Can you work these out from the drawing? Everything is in mm from the part's minimum corner. Give positions to 0.01 mm unless a question says otherwise; leave off trailing zeros. Order: outer loops, then holes, each group sorted by start corner. A loop starts at its lowest first (then second) coordinate and runs counter-clockwise, first axis right, second up. Notation, with made-up numbers: (-2.75, 45) - (53.25, 45) arc R10 ccw to (53.25, 50) - close; hole circle Ø2 at (-23.75, 0.5). An arc over 180 degrees is marked (long way). One line per question, with ' | ' between items.
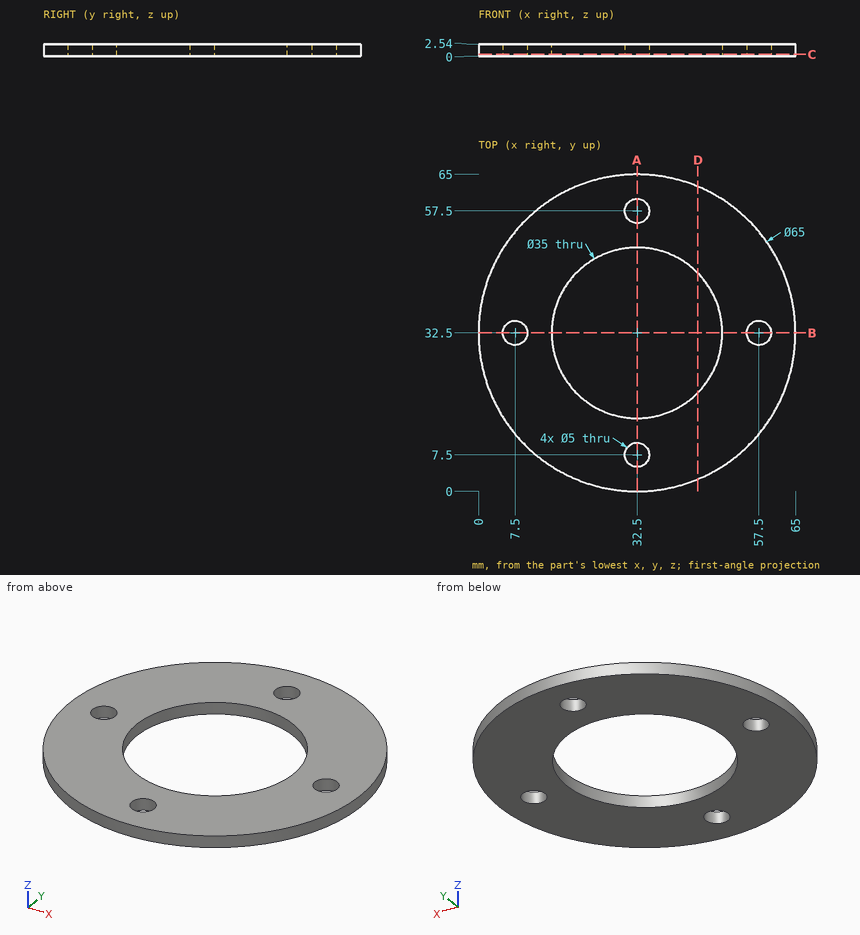
1) Please list where these lines run through material, in increasing order: L1, parallel to Y at x = 32.5, z = 2.05; L2, parallel to Y at x = 30.5, z = 1.65; L3, parallel to Y at x = 57.5, z = 0.55.
Model answer:
L1: y = 0 to 5, 10 to 15, 50 to 55, 60 to 65 | L2: y = 0.06 to 6, 9 to 15.11, 49.89 to 56, 59 to 64.94 | L3: y = 11.73 to 30, 35 to 53.27
2) I'm going to push a flat-ended pin straight in: P1, Ø1.5, axis at x = 39.5, z = 1.5, coming from the +Y side. Where does the tip first touch, or does it pass through?
Model answer:
P1: stops at y = 64.39
3) I want a section at A-A (x = 32.5). List the corners of the cut face in (y, z) for me, plus the area to 3 significant figures.
Model answer:
outline: (0, 0) - (5, 0) - (5, 2.54) - (0, 2.54) - close; (10, 0) - (15, 0) - (15, 2.54) - (10, 2.54) - close; (50, 0) - (55, 0) - (55, 2.54) - (50, 2.54) - close; (60, 0) - (65, 0) - (65, 2.54) - (60, 2.54) - close | area: 50.8 mm2
4) I want a section at C-C (z = 0.4). List the corners of the cut face in (x, y) for me.
Model answer:
outline: circle Ø65 at (32.5, 32.5); hole circle Ø5 at (7.5, 32.5); hole circle Ø35 at (32.5, 32.5); hole circle Ø5 at (32.5, 7.5); hole circle Ø5 at (32.5, 57.5); hole circle Ø5 at (57.5, 32.5)
5) I want a section at D-D (x = 45). List the corners of the cut face in (y, z) for me, plus the area to 3 significant figures.
Model answer:
outline: (2.5, 0) - (20.25, 0) - (20.25, 2.54) - (2.5, 2.54) - close; (44.75, 0) - (62.5, 0) - (62.5, 2.54) - (44.75, 2.54) - close | area: 90.2 mm2
